For this review, take the finished solid that the model builds, in its own axes (mm). A direction names the side the tool comes from. Round coordinates to 2 decimals unless told otherwise and drop trailing zeros. Write each loop counter-clockwise with the first axis right and the second up, starting at its lowest first coordinate (ties: lowest second). Pieces come first, ordered by that corner, then holes.
from build123d import *

# Parameters (mm, degrees)
SKETCH_1_R      = 5
SKETCH_1_R_2    = 2.5
EXTRUDE_1_DEPTH = 3.4
SKETCH_2_R      = 5
EXTRUDE_2_DEPTH = 1.9


with BuildPart() as part:
    # 草图1 → 凸台-拉伸1 (new, symmetric)
    with BuildSketch(Plane(origin=(0, 0, 0), x_dir=(1, 0, 0), z_dir=(0, 1, 0))):
        with Locations(Location((0, 0, 0), (0, 0, 270))):
            Circle(SKETCH_1_R)
        with Locations(Location((0, 0, 0), (0, 0, 270))):
            Circle(SKETCH_1_R_2, mode=Mode.SUBTRACT)
    extrude(amount=EXTRUDE_1_DEPTH, both=True)

    # 草图2 → 凸台-拉伸2 (add, symmetric)
    with BuildSketch(Plane(origin=(0, 0, 0), x_dir=(1, 0, 0), z_dir=(0, 1, 0))):
        Polygon((5, 3.002496099), (5, 75), (-5, 75), (-5, 3.002496099), (-67.351667387, -32.996255851), (-62.351667387, -41.656509889), (0, -5.657757939), (62.351667387, -41.656509889), (67.351667387, -32.996255851), align=None)
        with Locations(Location((0, 0, 0), (0, 0, 270))):
            Circle(SKETCH_2_R, mode=Mode.SUBTRACT)
    extrude(amount=EXTRUDE_2_DEPTH, both=True)


solid = part.part
(1) We need section C-C, the plane z = -30.5. Give the boundary of the cut face in (x, y).
Geometry check:
outline: (-5, -1.9) - (5, -1.9) - (5, 1.9) - (-5, 1.9) - close
(2) For faces 1 (the face through (5, 0, -38)), 2 (the face through (-4.88, -2.64, -1.08)), 3 (the face through (30.739, 0.027, 23.405)), 4 (the face through (-4.88, 2.66, -1.08)), 5 (the face through (-2, -3.4, 2)), list the 3-axis set-ups (+Z, -Z, +X, -X, +Y, -Y) from which the entire face can be reached by the end or side of a thin tool; tool diameter is ignored.
Geometry check:
face 1: -Z, +X, +Y, -Y
face 2: -Y
face 3: +Z, +Y, -Y
face 4: +Y
face 5: +Z, -Z, +X, -X, -Y
(3) For pin 1 Ø1 at (x, y) = (0.5, 2.5) entering from -Z; pin 2 Ø1.9 at (y, z) = (1, -25.5) entering from -X; pin 3 Ø1.5 at (x, y) = (-16.5, -2.5) entering from +Z, all flat-tipped, find the tip position at first contact; note any pin that passes through.
Geometry check:
pin 1: stops at z = -5
pin 2: stops at x = -5
pin 3: stops at z = 15.44
(4) We need section B-B, the plane z = 0. Give the boundary of the cut face in (x, y).
Geometry check:
outline: (-10.2, -1.9) - (-5, -1.9) - (-5, -3.4) - (-2.5, -3.4) - (-2.5, 3.4) - (-5, 3.4) - (-5, 1.9) - (-10.2, 1.9) - close; (2.5, -3.4) - (5, -3.4) - (5, -1.9) - (10.2, -1.9) - (10.2, 1.9) - (5, 1.9) - (5, 3.4) - (2.5, 3.4) - close
(5) For line 1 along Y through (x, z) = (43.5, 26.5); line 2 along X through (y, z) = (1.5, -14); line 3 along X through (y, z) = (0.5, 0), list the stretches that pass through material, from the lowest coordinate up.
Geometry check:
line 1: y = -1.9 to 1.9
line 2: x = -5 to 5
line 3: x = -10.2 to -2.5, 2.5 to 10.2
(6) We need section A-A, the plane y = 0.5. Give the boundary of the cut face in (x, z), and give its area (3 significant figures).
Geometry check:
outline: (-67.35, 33) - (-5, -3) - (-5, -75) - (5, -75) - (5, -3) - (67.35, 33) - (62.35, 41.66) - (0, 5.66) - (-62.35, 41.66) - close; hole circle Ø5 at (0, 0)
area: 2,180 mm2
(7) Mouldability with a two-part tool opening along Z and no side actions: class faces 6 (the face through (0, 0, -75)), 7 (the face through (-5, 0, -40)), 8 (the face through (64.817, 0.027, 37.387)), 9 (the face through (-2.44, -0.05, -0.54)) as pulls with the +Z half, pulls with the -Z half, needs draft (parallel to the pull), parting line crosses it, or undercut.
Geometry check:
face 6: pulls with the -Z half
face 7: needs draft
face 8: pulls with the +Z half
face 9: undercut
(8) We need section D-D, the plane x = -17. Give the boundary of the cut face in (y, z).
Geometry check:
outline: (-1.9, 3.93) - (1.9, 3.93) - (1.9, 15.47) - (-1.9, 15.47) - close
